Can you work these out from the model? Positions are in its coordinate system, mm. Face numbers are marked on the shaded views. Round coordinates to 2 decimals unless told otherwise and drop trailing zeros. Write each loop counter-clockwise with the first axis right and the second up, starting at its lowest first coordinate (ties: lowest second). Pieces come first, ordered by that corner, then holes. Notation, with made-up numbers: M -24,5 L 21,5 A15 ccw 21,31 Z; hole C 46.5,-1.75 d2. An arc over 180 degrees is marked long. Answer as a JSON object with one key per item and string values. Group by question number.
1) Suppose I cut it at C-C, the plane x = 25. Write out the boundary of the cut face in (y, z), and give its area (3 significant figures).
2) Suppose I cut it at A-A, the plane y = 14.5. Write out the boundary of the cut face in (x, z) (1 decimal), and give its area (3 significant figures).
3) Suppose I cut it at B-B, the plane z = -1. Write out the boundary of the cut face in (x, y) (1 decimal), and give its area (3 significant figures).
4) I'm going to push a flat-ended pin straight in: pin 1 Ø5.5 at (x, z) = (-2.24, -10.89) entering from -Y. Where does the tip first touch, or does it pass through?
5) If we mould it in two halves opening along X, with no side actions, what happens to the marked faces 1, 2, 3 and 4? For each: +X half, -X half, draft (parallel to the pull), parting line (faces both ways), or undercut.
6) Suppose I cut it at D-D, the plane z = -8.5. Write out the boundary of the cut face in (x, y) (1 decimal).
7) Please list where these lines run through material, in increasing order: L1, parallel to Z at x = 0, y = 60; L2, parallel to X at y = 43, z = -1.5; L3, parallel to Z at x = -1.5, y = 15.5. Write a range as [from, to].
from build123d import *

# Parameters (mm, degrees)
SKETCH3_W           = 76.2
SKETCH3_H           = 50.8
BOSS_EXTRUDE1_DEPTH = 76.2
SKETCH5_R           = 4.1275
CUT_EXTRUDE1_DEPTH  = 76.2
SKETCH6_R           = 4.445
CUT_EXTRUDE2_DEPTH  = 76.2
SKETCH8_R           = 4.445
CUT_EXTRUDE4_DEPTH  = 76.2
SKETCH9_R           = 4.445
CUT_EXTRUDE5_DEPTH  = 76.2
SKETCH10_R          = 4.445
CUT_EXTRUDE6_DEPTH  = 76.2
SKETCH12_R          = 4.7625
CUT_EXTRUDE7_DEPTH  = 76.2
SKETCH13_R          = 4.7625
CUT_EXTRUDE8_DEPTH  = 76.2


with BuildPart() as part:
    # Sketch3 → Boss-Extrude1 (new body)
    with BuildSketch(Plane(origin=(0, 0, 0), x_dir=(1, 0, 0), z_dir=(0, 1, 0))):
        with Locations((-2.241176471, -1.805392157)):
            Rectangle(SKETCH3_W, SKETCH3_H)
    extrude(amount=BOSS_EXTRUDE1_DEPTH)

    # Sketch5 → Cut-Extrude1 (cut)
    with BuildSketch(Plane(origin=(0, 76.2, 0), x_dir=(1, 0, 0), z_dir=(0, 1, 0))):
        with Locations(Location((-2.241176471, -1.805392157, 0), (0, 0, 270))):
            Circle(SKETCH5_R)
    extrude(amount=-CUT_EXTRUDE1_DEPTH, mode=Mode.SUBTRACT)

    # Sketch6 → Cut-Extrude2 (cut)
    with BuildSketch(Plane(origin=(0, 76.2, 0), x_dir=(1, 0, 0), z_dir=(0, 1, 0))):
        with Locations(Location((-14.941176471, -1.805392157, 0), (0, 0, 270))):
            Circle(SKETCH6_R)
    extrude(amount=-CUT_EXTRUDE2_DEPTH, mode=Mode.SUBTRACT)

    # Sketch8 → Cut-Extrude4 (cut)
    with BuildSketch(Plane(origin=(0, 76.2, 0), x_dir=(1, 0, 0), z_dir=(0, 1, 0))):
        with Locations(Location((10.458823529, -1.805392157, 0), (0, 0, 270))):
            Circle(SKETCH8_R)
    extrude(amount=-CUT_EXTRUDE4_DEPTH, mode=Mode.SUBTRACT)

    # Sketch9 → Cut-Extrude5 (cut)
    with BuildSketch(Plane(origin=(0, 76.2, 0), x_dir=(1, 0, 0), z_dir=(0, 1, 0))):
        with Locations(Location((-2.241176471, -14.505392157, 0), (0, 0, 270))):
            Circle(SKETCH9_R)
    extrude(amount=-CUT_EXTRUDE5_DEPTH, mode=Mode.SUBTRACT)

    # Sketch10 → Cut-Extrude6 (cut)
    with BuildSketch(Plane(origin=(0, 76.2, 0), x_dir=(1, 0, 0), z_dir=(0, 1, 0))):
        with Locations(Location((-2.241176471, 10.894607843, 0), (0, 0, 270))):
            Circle(SKETCH10_R)
    extrude(amount=-CUT_EXTRUDE6_DEPTH, mode=Mode.SUBTRACT)

    # Sketch12 → Cut-Extrude7 (cut)
    with BuildSketch(Plane.XY.offset(27.205392157)):
        with Locations((-29.241376471, 62.5602)):
            Circle(SKETCH12_R)
    extrude(amount=-CUT_EXTRUDE7_DEPTH, mode=Mode.SUBTRACT)

    # Sketch13 → Cut-Extrude8 (cut)
    with BuildSketch(Plane.XY.offset(27.205392157)):
        with Locations((22.219023529, 11.0998)):
            Circle(SKETCH13_R)
    extrude(amount=-CUT_EXTRUDE8_DEPTH, mode=Mode.SUBTRACT)


solid = part.part
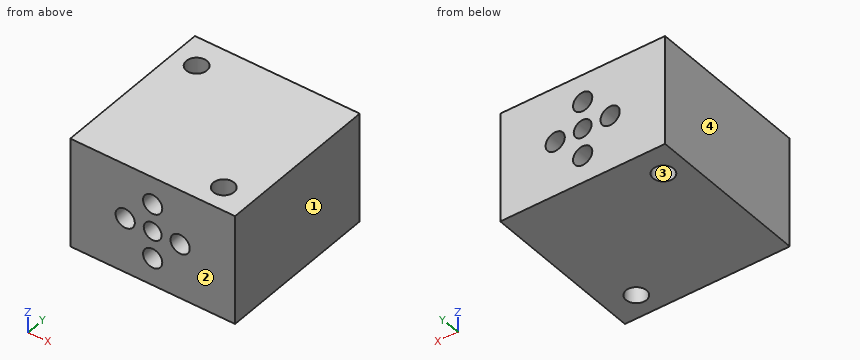
Results:
{
 "1": {"outline": "M 0,-23.59 L 7.23,-23.59 L 7.23,27.21 L 0,27.21 Z; M 14.97,-23.59 L 76.2,-23.59 L 76.2,27.21 L 14.97,27.21 Z", "area": "3,480 mm^2"},
 "2": {"outline": "M -40.3,-23.6 L 18.9,-23.6 L 18.9,27.2 L -40.3,27.2 Z; M 25.6,-23.6 L 35.9,-23.6 L 35.9,27.2 L 25.6,27.2 Z; hole C -14.9,1.8 d8.9; hole C -2.2,-10.9 d8.9; hole C -2.2,14.5 d8.9; hole C -2.2,1.8 d8.3; hole C 10.5,1.8 d8.9", "area": "3,230 mm^2"},
 "3": {"outline": "M -40.3,0 L -18.4,0 L -18.4,76.2 L -40.3,76.2 Z; M -11.5,0 L -5.3,0 L -5.3,76.2 L -11.5,76.2 Z; M 0.8,0 L 7,0 L 7,76.2 L 0.8,76.2 Z; M 13.9,0 L 35.9,0 L 35.9,76.2 L 13.9,76.2 Z; hole C -29.2,62.6 d9.5; hole C 22.2,11.1 d9.5", "area": "4,150 mm^2"},
 "4": {"pin 1": "through"},
 "5": {"face 1": "+X half", "face 2": "draft", "face 3": "undercut", "face 4": "-X half"},
 "6": {"outline": "M -40.3,0 L -6,0 L -6,76.2 L -40.3,76.2 Z; M 1.5,0 L 35.9,0 L 35.9,76.2 L 1.5,76.2 Z; hole C -29.2,62.6 d9.5; hole C 22.2,11.1 d9.5"},
 "7": {"L1": "[-23.59, -14.73], [-7.06, -1.66], [5.27, 10.67], [18.34, 27.21]", "L2": "[-40.34, -17.91], [-11.97, -4.71], [0.23, 7.49], [13.43, 35.86]", "L3": "[-23.59, -15.28], [-6.51, -2.26], [5.87, 10.12], [18.89, 27.21]"}
}
